from build123d import *

# Parameters (mm, degrees)
SKETCH_1_R      = 6
SKETCH_1_R_2    = 3
EXTRUDE_1_DEPTH = 8
SKETCH_2_R      = 9
SKETCH_2_R_2    = 3
EXTRUDE_2_DEPTH = 4
SKETCH_3_R      = 4
SKETCH_3_R_2    = 2
EXTRUDE_3_DEPTH = 15
CHAMFER_1_SIZE  = 2
CHAMFER_2_SIZE  = 3
CHAMFER_2_SIZE2 = 1
FILLET_1_R      = 1
SKETCH_4_R      = 9
SKETCH_4_R_2    = 2.15
EXTRUDE_5_DEPTH = 3


with BuildPart() as part:
    # 草图1 → 凸台-拉伸1 (new body)
    with BuildSketch(Plane.XY):
        Circle(SKETCH_1_R)
        Circle(SKETCH_1_R_2, mode=Mode.SUBTRACT)
    extrude(amount=EXTRUDE_1_DEPTH)

    # 草图2 → 凸台-拉伸2 (add)
    with BuildSketch(Plane.XY.offset(8)):
        Circle(SKETCH_2_R)
        Circle(SKETCH_2_R_2, mode=Mode.SUBTRACT)
    extrude(amount=EXTRUDE_2_DEPTH)

    # 草图3 → 凸台-拉伸3 (add)
    with BuildSketch(Plane.XY.offset(12)):
        Circle(SKETCH_3_R)
        Circle(SKETCH_3_R_2, mode=Mode.SUBTRACT)
    extrude(amount=EXTRUDE_3_DEPTH)

    # 倒角1
    # the kernel refuses this chamfer: 2 mm, written as the material it adds along each edge
    with BuildSketch(Plane(origin=(0, 0, 12), x_dir=(1, 0, 0), z_dir=(0, -1, 0))) as chamfer_1_piece_1:
        Polygon((4 + CHAMFER_1_SIZE, 0), (4, CHAMFER_1_SIZE), (4, 0), align=None)
    revolve(axis=Axis((0, 0, 12), (0, 0, 1)))
    # the kernel refuses this chamfer: 2 mm, written as the material it takes off along each edge
    with BuildSketch(Plane(origin=(0, 0, 12), x_dir=(1, 0, 0), z_dir=(0, -1, 0))) as chamfer_1_2_piece_1_section:
        Polygon((2 + CHAMFER_1_SIZE, 0), (2, CHAMFER_1_SIZE), (2, 0), align=None)
    chamfer_1_2_piece_1 = revolve(axis=Axis((0, 0, 12), (0, 0, 1)), mode=Mode.PRIVATE)
    chamfer_1_2_piece_1 = chamfer_1_2_piece_1 & Plane(origin=(0, 0, 13.507652587), x_dir=(1, 0, 0), z_dir=(0, 0, -1)) * Cylinder(3, 16, mode=Mode.PRIVATE)
    add(chamfer_1_2_piece_1, mode=Mode.SUBTRACT)

    # 倒角2
    chamfer_2_edges = [part.edges().sort_by_distance(p)[0] for p in [
        (-4, 0, 27),
    ]]
    chamfer_2_side = [part.faces().sort_by_distance(p)[0] for p in [
        (-4, 0, 20.5),
    ]]
    chamfer(chamfer_2_edges, length=CHAMFER_2_SIZE, length2=CHAMFER_2_SIZE2, reference=chamfer_2_side[0])

    # 圆角1
    fillet_1_edges = [part.edges().sort_by_distance(p)[0] for p in [
        (-3, 0, 27),
        (-4, 0, 24),
    ]]
    fillet(fillet_1_edges, radius=FILLET_1_R)

    # 草图4 → 凸台-拉伸5 (add)
    with BuildSketch(Plane.XY.offset(8)):
        with BuildLine():
            Line((-22.7, 5.35817133), (-6.75, 13.395428325))
            ThreePointArc((-6.75, 13.395428325), (0, 15), (6.75, 13.395428325))
            Line((6.75, 13.395428325), (22.7, 5.35817133))
            ThreePointArc((22.7, 5.35817133), (26, 0), (22.7, -5.35817133))
            Line((22.7, -5.35817133), (6.75, -13.395428325))
            ThreePointArc((6.75, -13.395428325), (0, -15), (-6.75, -13.395428325))
            Line((-6.75, -13.395428325), (-22.7, -5.35817133))
            ThreePointArc((-22.7, -5.35817133), (-26, 0), (-22.7, 5.35817133))
        make_face()
        Circle(SKETCH_4_R, mode=Mode.SUBTRACT)
        with Locations((20, 0)):
            Circle(SKETCH_4_R_2, mode=Mode.SUBTRACT)
        with Locations((-20, 0)):
            Circle(SKETCH_4_R_2, mode=Mode.SUBTRACT)
    extrude(amount=EXTRUDE_5_DEPTH)


solid = part.part
For this review, take the finished solid that the model builds, in its own axes (mm). A direction names the side the tool comes from. Round coordinates to 2 decimals unless told otherwise and drop trailing zeros. Loops run counter-clockwise (first coordinate to the right, second up) from the corner with the lowest first, then second, coordinate; pieces in that order, holes last. Notation, with made-up numbers: (-13.5, 83) - (30.5, 83) arc R20 ccw to (30.5, 114) - close; hole circle Ø4 at (-7, 64). An arc over 180 degrees is marked (long way). Put each result on its own line as item: value. Start each with the question number.
1. For probe 1 along Z at (x, y) = (-8, -5); probe 2 along Y at (x, z) = (-20, 8.9); probe 3 along Y at (x, z) = (0, 4.75), list the stretches that pass through material, from the lowest coordinate up. Write a range as [from, to].
2. Consider section A-A on z = 9.5. State the section outline as (x, y) points.
3. Insertion check: P1, Ø1.5, axis at x = -8.5, y = 2, coming from the -Z side; P2, Ø8, axis at x = 20.5, y = 0.5, coming from the +Z side; P3, Ø4, axis at y = -4, z = 4, coming from the +X side. Each pin has a flat end and moves straight along its axis. Give the tip position at first contact, or say it passes through.
4. Consider section D-D on x = -20. State the section outline as (y, z) points.
5. For faces 1 (the cylindrical face through (3.695, -1.532, 18.85)), 2 (the flat face through (6, 4, 8)), 3 (the flat face through (14.613, 9.433, 9.479)), list the 3-axis set-ups (+Z, -Z, +X, -X, +Y, -Y) from which the entire face can be reached by the end or side of a thin tool; tool diameter is ignored.
6. Consider section B-B on x = 19. State the section outline as (y, z) points.
7. Consider section C-C on y = 0. State how many separate pieces and enclosed holes the cut face has, plus the area to 3 significant figures.
8. Mouldability with a two-part tool opening along Y and no side actions: class faces 4 (the cylindrical face through (0, 15, 9)), 5 (the cylindrical face through (-6, 0, 4)), 6 (the cylindrical face through (-22.15, 0.09, 9.48)), 7 (the flat face through (14.84, -9.32, 9.48)) as +Y half, -Y half, draft (parallel to the pull), parting line (faces both ways), or undercut.
Result sheet:
1. probe 1: [8, 11]
1. probe 2: [-6.72, -2.15], [2.15, 6.72]
1. probe 3: [-6, -3], [3, 6]
2. outline: (-22.7, -5.36) - (-6.75, -13.4) arc R15 ccw to (6.75, -13.4) - (22.7, -5.36) arc R6 ccw to (22.7, 5.36) - (6.75, 13.4) arc R15 ccw to (-6.75, 13.4) - (-22.7, 5.36) arc R6 ccw to start; hole circle Ø4.3 at (-20, 0); hole circle Ø6 at (0, 0); hole circle Ø4.3 at (20, 0)
3. P1: z = 8
3. P2: z = 11
3. P3: x = 5.66
4. outline: (-6.72, 8) - (-2.15, 8) - (-2.15, 11) - (-6.72, 11) - close; (2.15, 8) - (6.72, 8) - (6.72, 11) - (2.15, 11) - close
5. face 1: +Z
5. face 2: -Z
5. face 3: +Z, -Z, +X, +Y
6. outline: (-7.22, 8) - (-1.9, 8) - (-1.9, 11) - (-7.22, 11) - close; (1.9, 8) - (7.22, 8) - (7.22, 11) - (1.9, 11) - close
7. separate pieces: 4
7. enclosed holes: 0
7. area: 230 mm^2
8. face 4: +Y half
8. face 5: parting line
8. face 6: undercut
8. face 7: -Y half
